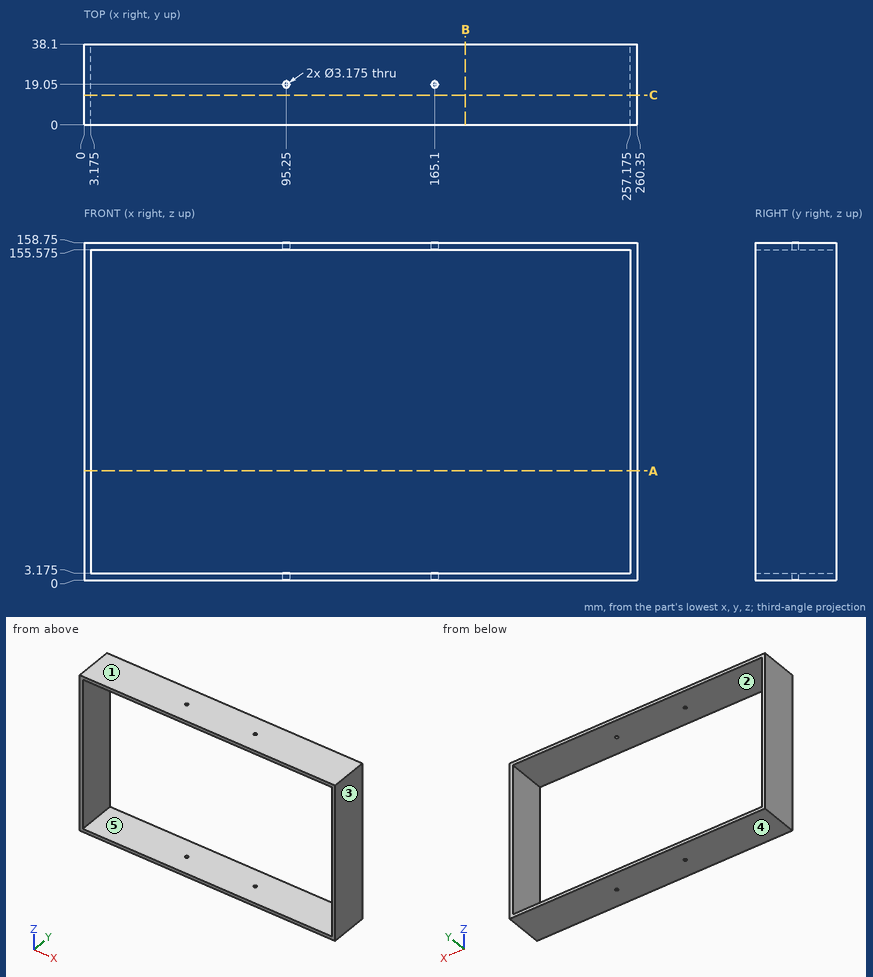
Drawing for the job (mm, zero at the part's lowest x, y, z). A direction names the side the tool comes from. Round coordinates to 2 decimals unless told otherwise and drop trailing zeros. Loops run counter-clockwise (first coordinate to the right, second up) from the corner with the lowest first, then second, coordinate; pieces in that order, holes last. Notation, with made-up numbers: (58.5, 48) - (106.5, 48) arc R9 ccw to (106.5, 64) - close; hole circle Ø8 at (10.5, 69.25). An arc over 180 degrees is marked (long way). Write each question's results on one line, items separated by ' | '.
(1) Wall check: L1, parallel to Z at x = 58, y = 8.5 (3 decimals); L2, parallel to X at y = 31, z = 58 (3 decimals); L3, parallel to Y at x = 95, z = 1. Give the ranges that are in metal, low to high.
Answer below:
L1: z = 0 to 3.175, 155.575 to 158.75 | L2: x = 0 to 3.175, 257.175 to 260.35 | L3: y = 0 to 17.48, 20.62 to 38.1
(2) 3-axis set-ups, long thin cutter, end or side, ignore diameter. For the marked faces 1 and 2: which of +Z, -Z, +X, -X, +Y, -Y reach the whole face in a straight line?
Answer below:
face 1: +Z, +X, -X, +Y, -Y | face 2: +Y, -Y
(3) Mould opens along Z. For the marked faces 3, 4 and 5 say: released by +Z, released by -Z, zero draft, split by the parting line, or undercut.
Answer below:
face 3: zero draft | face 4: released by -Z | face 5: undercut
(4) Saw through at A-A, the plane z = 51.5. List the corners of the cut face in (x, y) (3 decimals).
Answer below:
outline: (0, 0) - (3.175, 0) - (3.175, 38.1) - (0, 38.1) - close; (257.175, 0) - (260.35, 0) - (260.35, 38.1) - (257.175, 38.1) - close
(5) Saw through at B-B, the plane x = 179.5. List the corners of the cut face in (y, z) (3 decimals), then the cut area to 3 significant figures.
Answer below:
outline: (0, 0) - (38.1, 0) - (38.1, 3.175) - (0, 3.175) - close; (0, 155.575) - (38.1, 155.575) - (38.1, 158.75) - (0, 158.75) - close | area: 242 mm^2
(6) Saw through at C-C, the plane y = 14. List the corners of the cut face in (x, z) (3 decimals), then the cut area to 3 significant figures.
Answer below:
outline: (0, 0) - (260.35, 0) - (260.35, 158.75) - (0, 158.75) - close; hole (3.175, 3.175) - (257.175, 3.175) - (257.175, 155.575) - (3.175, 155.575) - close | area: 2,620 mm^2
(7) Pin check, flat tip, straight feed: pin 1 (2.5 mm diameter, centred on x = 95.25, y = 19.05, fed in from +Z). Stop position of the tip, or through.
Answer below:
pin 1: passes through
